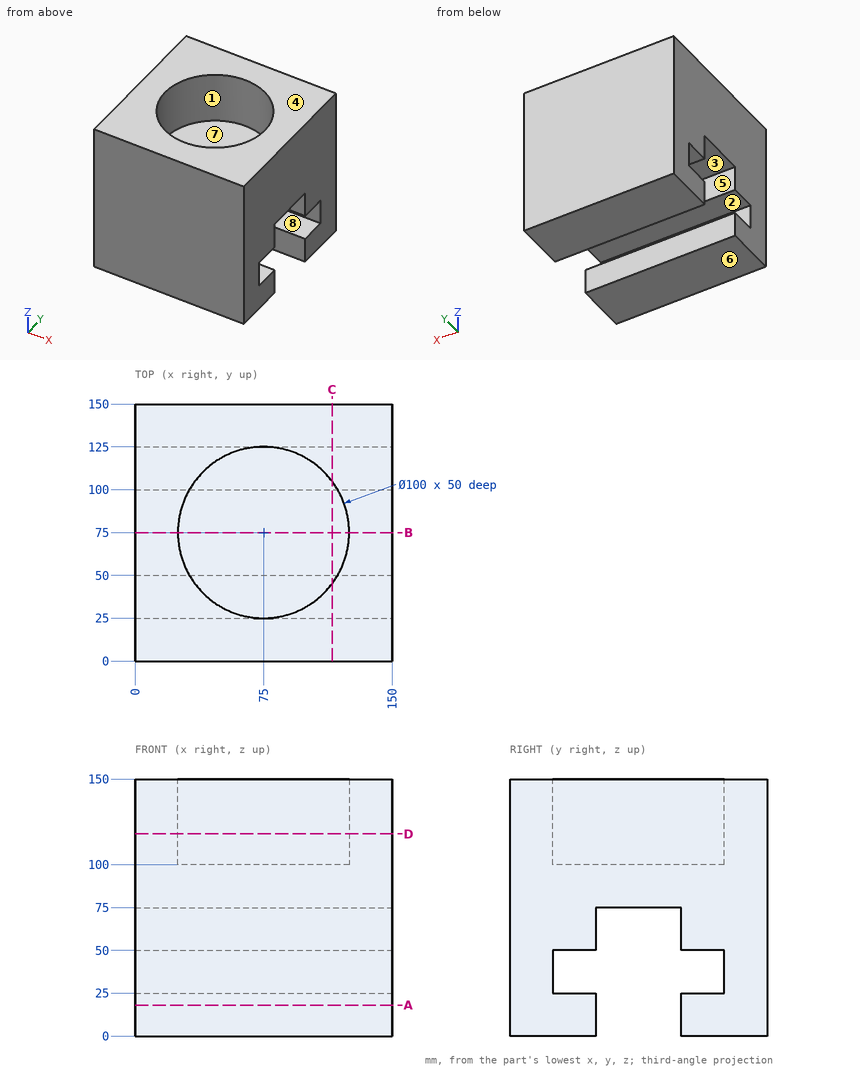
Geometry: see drawing. Coordinates: mm, zero at the bounding-box minimum. A direction names the side the tool comes from. Coordinates: 2 decimals unless noted, no trailing zeros. Write each loop counter-clockwise with the first axis right and the second up, starting at its lowest first coordinate (ties: lowest second). Pieces come first, ordered by that corner, then holes. Notation, with made-up numbers: (40, 19.5) - (83, 19.5) arc R23 ccw to (83, 49.5) - close; hole circle Ø3 at (14, 72.25). An arc over 180 degrees is marked (long way). Put each result on its own line as item: value. Start each with the question number.
1) Cut plane C-C (x = 115). Return the cut outline in (y, z).
2) Contact query for flat-ended pins moving along their axis: pin 1 (1 mm diameter, centred on x = 134, z = 53, fed in from -Y); pin 2 (1.5 mm diameter, centred on x = 64, y = 117.5, fed in from +Z). Output: stop coordinate, or through.
3) Cut plane B-B (y = 75). Return the cut outline in (x, z), plus the area to 3 significant figures.
4) Cut plane A-A (z = 18). Return the cut outline in (x, y).
5) Cut plane D-D (z = 118). Return the cut outline in (x, y), plus the area to 3 significant figures.
6) Reachability of the marked faces 1, 2, 3 and 4 from +Z, -Z, +X, -X, +Y, -Y: full face, straight path, thin tool, end or side. Return the list, or none.
7) Mould query, pull axis Z, two halves, no side actions, for the marked faces 5, 6, 7 and 8. Classes: pulls with the +Z half, pulls with the -Z half, needs draft (parallel to the pull), parting line crosses it, or undercut.
8) Ray query, L1, parallel to Y at x = 30, z = 11; L2, parallel to Y at x = 14, z = 43; L3, parallel to Z at x = 97, y = 113. Return the intervals inside material, ascending.
Resolved:
1. outline: (0, 0) - (50, 0) - (50, 25) - (25, 25) - (25, 50) - (50, 50) - (50, 75) - (100, 75) - (100, 50) - (125, 50) - (125, 25) - (100, 25) - (100, 0) - (150, 0) - (150, 150) - (105, 150) - (105, 100) - (45, 100) - (45, 150) - (0, 150) - close
2. pin 1: stops at y = 0
2. pin 2: stops at z = 100
3. outline: (0, 75) - (150, 75) - (150, 150) - (125, 150) - (125, 100) - (25, 100) - (25, 150) - (0, 150) - close
3. area: 6,250 mm2
4. outline: (0, 0) - (150, 0) - (150, 50) - (0, 50) - close; (0, 100) - (150, 100) - (150, 150) - (0, 150) - close
5. outline: (0, 0) - (150, 0) - (150, 150) - (0, 150) - close; hole circle Ø100 at (75, 75)
5. area: 14,600 mm2
6. face 1: +Z
6. face 2: +X, -X
6. face 3: -Z, +X, -X
6. face 4: +Z, +X, -X, +Y, -Y
7. face 5: needs draft
7. face 6: pulls with the -Z half
7. face 7: pulls with the +Z half
7. face 8: undercut
8. L1: y = 0 to 50, 100 to 150
8. L2: y = 0 to 25, 125 to 150
8. L3: z = 0 to 25, 50 to 100
